Geometry check sheet. Reference: the model listing, model coordinates, mm. A direction names the side the tool comes from. Give positions to 0.01 mm unless a question says otherwise; leave off trailing zeros. Write each loop counter-clockwise with the first axis right and the second up, starting at its lowest first coordinate (ties: lowest second). Pieces come first, ordered by that corner, then holes. Notation, with made-up numbers: (-2.5, 9) -> (16.5, 9) arc R26 cw to (16.5, 47) -> close; hole circle Ø8 at (5.25, 16.5). An arc over 180 degrees is marked (long way). One line per item, written item: value.
from build123d import *

# Parameters (mm, degrees)
F0_W         = 88.9
F0_H         = 88.9
F0_W_2       = 57.15
F0_H_2       = 57.15
F1_DEPTH     = 177.8
F2_DEPTH     = 15.875
F3_R         = 3.429
F4_T1_DEPTH  = 57.15
F4_T3_DEPTH  = 57.15
F4_T9_DEPTH  = 97.975467434
F4_T13_DEPTH = 97.975467434
F4_T20_DEPTH = 97.975467434
F4_T24_DEPTH = 97.975467434
F4_T31_DEPTH = 97.975467434
F4_T35_DEPTH = 97.975467434
F4_T42_DEPTH = 97.975467434
F4_T46_DEPTH = 97.975467434


# Not quite as in the source:
# - a fillet or chamfer that OpenCascade refuses, or shapes differently, is made with other operations: its cross-section is extruded or revolved along the edge and cut away or added


with BuildPart() as f1:
    # F0 (on Front) → F1 (new body)
    with BuildSketch(Plane.XZ):
        Rectangle(F0_W, F0_H)
        Rectangle(F0_W_2, F0_H_2, mode=Mode.SUBTRACT)
    extrude(amount=-F1_DEPTH)

    # F0 (on Front) → F2 (join)
    with BuildSketch(Plane.XZ):
        Rectangle(F0_W, F0_H)
        Rectangle(F0_W_2, F0_H_2, mode=Mode.SUBTRACT)
        Rectangle(F0_W_2, F0_H_2)
    extrude(amount=-F2_DEPTH)

    # F3
    f3_edges = [f1.edges().sort_by_distance(p)[0] for p in [
        (44.45, 88.9, 44.45),
        (0, 0, 44.45),
        (44.45, 0, 0),
        (0, 0, -44.45),
        (44.45, 88.9, -44.45),
        (-44.45, 0, 0),
        (-44.45, 88.9, -44.45),
        (0, 177.8, 44.45),
        (-44.45, 88.9, 44.45),
        (-44.45, 177.8, 0),
        (0, 177.8, -44.45),
        (44.45, 177.8, 0),
    ]]
    fillet(f3_edges, radius=F3_R)

    # F4: chamfer of 15.875 on 4 edges, made by hand

    # F4_s2 → F4_t1 (cut)
    with BuildSketch(Plane.XY.offset(-28.575)):
        with BuildLine():
            Line((-44.8990128061, 178.2490128061), (-28.1259871939, 161.4759871939))
            Line((-28.1259871939, 161.4759871939), (-27.8084871939, 161.4759871939))
            ThreePointArc((-27.8084871939, 161.4759871939), (-28.2575, 169.637993597), (-28.2575, 177.8))
            Line((-28.2575, 177.8), (-28.575, 178.1175))
            ThreePointArc((-28.575, 178.1175), (-36.737006403, 178.1175), (-44.8990128061, 178.5665128061))
            Line((-44.8990128061, 178.5665128061), (-44.8990128061, 178.2490128061))
        make_face()
        with BuildLine():
            Line((44.8990128061, 178.2490128061), (28.1259871939, 161.4759871939))
            Line((28.1259871939, 161.4759871939), (27.8084871939, 161.4759871939))
            ThreePointArc((27.8084871939, 161.4759871939), (28.2575, 169.637993597), (28.2575, 177.8))
            Line((28.2575, 177.8), (28.575, 178.1175))
            ThreePointArc((28.575, 178.1175), (36.737006403, 178.1175), (44.8990128061, 178.5665128061))
            Line((44.8990128061, 178.5665128061), (44.8990128061, 178.2490128061))
        make_face()
    extrude(amount=F4_T1_DEPTH, mode=Mode.SUBTRACT)

    # F4_s4 → F4_t3 (cut)
    with BuildSketch(Plane.YZ.offset(-28.575)):
        with BuildLine():
            Line((178.2490128061, -44.8990128061), (161.4759871939, -28.1259871939))
            Line((161.4759871939, -28.1259871939), (161.4759871939, -27.8084871939))
            ThreePointArc((161.4759871939, -27.8084871939), (169.637993597, -28.2575), (177.8, -28.2575))
            Line((177.8, -28.2575), (178.1175, -28.575))
            ThreePointArc((178.1175, -28.575), (178.1175, -36.737006403), (178.5665128061, -44.8990128061))
            Line((178.5665128061, -44.8990128061), (178.2490128061, -44.8990128061))
        make_face()
        with BuildLine():
            Line((178.2490128061, 44.8990128061), (161.4759871939, 28.1259871939))
            Line((161.4759871939, 28.1259871939), (161.4759871939, 27.8084871939))
            ThreePointArc((161.4759871939, 27.8084871939), (169.637993597, 28.2575), (177.8, 28.2575))
            Line((177.8, 28.2575), (178.1175, 28.575))
            ThreePointArc((178.1175, 28.575), (178.1175, 36.737006403), (178.5665128061, 44.8990128061))
            Line((178.5665128061, 44.8990128061), (178.2490128061, 44.8990128061))
        make_face()
    extrude(amount=F4_T3_DEPTH, mode=Mode.SUBTRACT)


with BuildPart() as f4_tool7:
    # F4_s8 → F4_t9 (new body)
    with BuildSketch(Plane.XY.offset(-69.400467434)):
        with BuildLine():
            Line((-44.8990128061, 178.2490128061), (-28.1259871939, 161.4759871939))
            Line((-28.1259871939, 161.4759871939), (-27.8084871939, 161.4759871939))
            ThreePointArc((-27.8084871939, 161.4759871939), (-28.2575, 169.637993597), (-28.2575, 177.8))
            Line((-28.2575, 177.8), (-28.575, 178.1175))
            ThreePointArc((-28.575, 178.1175), (-36.737006403, 178.1175), (-44.8990128061, 178.5665128061))
            Line((-44.8990128061, 178.5665128061), (-44.8990128061, 178.2490128061))
        make_face()
    extrude(amount=F4_T9_DEPTH)

    split(bisect_by=Plane.XY.offset(-28.575), keep=Keep.BOTTOM)


with BuildPart() as f4_tool11:
    # F4_s12 → F4_t13 (new body)
    with BuildSketch(Plane.YZ.offset(28.575)):
        with BuildLine():
            Line((178.2490128061, -44.8990128061), (161.4759871939, -28.1259871939))
            Line((161.4759871939, -28.1259871939), (161.4759871939, -27.8084871939))
            ThreePointArc((161.4759871939, -27.8084871939), (169.637993597, -28.2575), (177.8, -28.2575))
            Line((177.8, -28.2575), (178.1175, -28.575))
            ThreePointArc((178.1175, -28.575), (178.1175, -36.737006403), (178.5665128061, -44.8990128061))
            Line((178.5665128061, -44.8990128061), (178.2490128061, -44.8990128061))
        make_face()
    extrude(amount=-F4_T13_DEPTH)

    split(bisect_by=Plane.YZ.offset(-28.575), keep=Keep.BOTTOM)


with BuildPart() as f4_tool7_1:
    add(f4_tool7.part)

    # F4_t15: intersect F4_tool11
    add(f4_tool11.part, mode=Mode.INTERSECT)


with BuildPart() as f1_1:
    add(f1.part)

    # F4_t5: cut F4_tool7
    add(f4_tool7_1.part, mode=Mode.SUBTRACT)


with BuildPart() as f4_tool18:
    # F4_s19 → F4_t20 (new body)
    with BuildSketch(Plane.XY.offset(-28.575)):
        with BuildLine():
            Line((-44.8990128061, 178.2490128061), (-28.1259871939, 161.4759871939))
            Line((-28.1259871939, 161.4759871939), (-27.8084871939, 161.4759871939))
            ThreePointArc((-27.8084871939, 161.4759871939), (-28.2575, 169.637993597), (-28.2575, 177.8))
            Line((-28.2575, 177.8), (-28.575, 178.1175))
            ThreePointArc((-28.575, 178.1175), (-36.737006403, 178.1175), (-44.8990128061, 178.5665128061))
            Line((-44.8990128061, 178.5665128061), (-44.8990128061, 178.2490128061))
        make_face()
    extrude(amount=F4_T20_DEPTH)

    split(bisect_by=Plane.XY.offset(28.575), keep=Keep.TOP)


with BuildPart() as f4_tool22:
    # F4_s23 → F4_t24 (new body)
    with BuildSketch(Plane.YZ.offset(-69.400467434)):
        with BuildLine():
            Line((178.2490128061, 44.8990128061), (161.4759871939, 28.1259871939))
            Line((161.4759871939, 28.1259871939), (161.4759871939, 27.8084871939))
            ThreePointArc((161.4759871939, 27.8084871939), (169.637993597, 28.2575), (177.8, 28.2575))
            Line((177.8, 28.2575), (178.1175, 28.575))
            ThreePointArc((178.1175, 28.575), (178.1175, 36.737006403), (178.5665128061, 44.8990128061))
            Line((178.5665128061, 44.8990128061), (178.2490128061, 44.8990128061))
        make_face()
    extrude(amount=F4_T24_DEPTH)

    split(bisect_by=Plane.YZ.offset(-28.575), keep=Keep.BOTTOM)


with BuildPart() as f4_tool18_1:
    add(f4_tool18.part)

    # F4_t26: intersect F4_tool22
    add(f4_tool22.part, mode=Mode.INTERSECT)


with BuildPart() as f1_2:
    add(f1_1.part)

    # F4_t16: cut F4_tool18
    add(f4_tool18_1.part, mode=Mode.SUBTRACT)


with BuildPart() as f4_tool29:
    # F4_s30 → F4_t31 (new body)
    with BuildSketch(Plane.XY.offset(28.575)):
        with BuildLine():
            Line((44.8990128061, 178.2490128061), (28.1259871939, 161.4759871939))
            Line((28.1259871939, 161.4759871939), (27.8084871939, 161.4759871939))
            ThreePointArc((27.8084871939, 161.4759871939), (28.2575, 169.637993597), (28.2575, 177.8))
            Line((28.2575, 177.8), (28.575, 178.1175))
            ThreePointArc((28.575, 178.1175), (36.737006403, 178.1175), (44.8990128061, 178.5665128061))
            Line((44.8990128061, 178.5665128061), (44.8990128061, 178.2490128061))
        make_face()
    extrude(amount=-F4_T31_DEPTH)

    split(bisect_by=Plane.XY.offset(-28.575), keep=Keep.BOTTOM)


with BuildPart() as f4_tool33:
    # F4_s34 → F4_t35 (new body)
    with BuildSketch(Plane.YZ.offset(69.400467434)):
        with BuildLine():
            Line((178.2490128061, -44.8990128061), (161.4759871939, -28.1259871939))
            Line((161.4759871939, -28.1259871939), (161.4759871939, -27.8084871939))
            ThreePointArc((161.4759871939, -27.8084871939), (169.637993597, -28.2575), (177.8, -28.2575))
            Line((177.8, -28.2575), (178.1175, -28.575))
            ThreePointArc((178.1175, -28.575), (178.1175, -36.737006403), (178.5665128061, -44.8990128061))
            Line((178.5665128061, -44.8990128061), (178.2490128061, -44.8990128061))
        make_face()
    extrude(amount=-F4_T35_DEPTH)

    split(bisect_by=Plane.YZ.offset(28.575), keep=Keep.TOP)


with BuildPart() as f4_tool29_1:
    add(f4_tool29.part)

    # F4_t37: intersect F4_tool33
    add(f4_tool33.part, mode=Mode.INTERSECT)


with BuildPart() as f1_3:
    add(f1_2.part)

    # F4_t27: cut F4_tool29
    add(f4_tool29_1.part, mode=Mode.SUBTRACT)


with BuildPart() as f4_tool40:
    # F4_s41 → F4_t42 (new body)
    with BuildSketch(Plane.YZ.offset(-28.575)):
        with BuildLine():
            Line((178.2490128061, 44.8990128061), (161.4759871939, 28.1259871939))
            Line((161.4759871939, 28.1259871939), (161.4759871939, 27.8084871939))
            ThreePointArc((161.4759871939, 27.8084871939), (169.637993597, 28.2575), (177.8, 28.2575))
            Line((177.8, 28.2575), (178.1175, 28.575))
            ThreePointArc((178.1175, 28.575), (178.1175, 36.737006403), (178.5665128061, 44.8990128061))
            Line((178.5665128061, 44.8990128061), (178.2490128061, 44.8990128061))
        make_face()
    extrude(amount=F4_T42_DEPTH)

    split(bisect_by=Plane.YZ.offset(28.575), keep=Keep.TOP)


with BuildPart() as f4_tool44:
    # F4_s45 → F4_t46 (new body)
    with BuildSketch(Plane.XY.offset(69.400467434)):
        with BuildLine():
            Line((44.8990128061, 178.2490128061), (28.1259871939, 161.4759871939))
            Line((28.1259871939, 161.4759871939), (27.8084871939, 161.4759871939))
            ThreePointArc((27.8084871939, 161.4759871939), (28.2575, 169.637993597), (28.2575, 177.8))
            Line((28.2575, 177.8), (28.575, 178.1175))
            ThreePointArc((28.575, 178.1175), (36.737006403, 178.1175), (44.8990128061, 178.5665128061))
            Line((44.8990128061, 178.5665128061), (44.8990128061, 178.2490128061))
        make_face()
    extrude(amount=-F4_T46_DEPTH)

    split(bisect_by=Plane.XY.offset(28.575), keep=Keep.TOP)


with BuildPart() as f4_tool40_1:
    add(f4_tool40.part)

    # F4_t48: intersect F4_tool44
    add(f4_tool44.part, mode=Mode.INTERSECT)


with BuildPart() as f1_4:
    add(f1_3.part)

    # F4_t38: cut F4_tool40
    add(f4_tool40_1.part, mode=Mode.SUBTRACT)


solid = f1_4.part
1) Mould release check, pull along X, two halves, no side actions. Record for faces 3 (the flat face through (-0.6, 169.46, 36.11)), 4 (the cylindrical face through (43.47, 1.03, 0.57)), 5 (the cylindrical face through (-43.47, 90.1, 43.42)), 6 (the flat face through (0.6, 169.46, -36.11)): released by +X, released by -X, zero draft, split by the parting line, or undercut.
Verdict:
face 3: undercut
face 4: released by +X
face 5: released by -X
face 6: undercut
2) Scan lines: probe 1 along Z at (x, y) = (18, 19.5) (3 decimals); probe 2 along X at (y, z) = (73.5, 41.5). Record each from-to range of solid material in increasing order.
Verdict:
probe 1: -44.45 to -28.575, 28.575 to 44.45
probe 2: -44.42 to 44.42
3) Sectioned sample at A-A on y = 129.5. Record the cut outline in (x, z) (3 decimals).
Verdict:
outline: (-44.45, -41.021) arc R3.429 ccw to (-41.021, -44.45) -> (41.021, -44.45) arc R3.429 ccw to (44.45, -41.021) -> (44.45, 41.021) arc R3.429 ccw to (41.021, 44.45) -> (-41.021, 44.45) arc R3.429 ccw to (-44.45, 41.021) -> close; hole (-28.575, -28.575) -> (28.575, -28.575) -> (28.575, 28.575) -> (-28.575, 28.575) -> close
4) Sectioned sample at C-C on x = 31.5. Record the cut outline in (y, z), plus the area to 3 significant figures.
Verdict:
outline: (0, -41.02) arc R3.43 ccw to (3.43, -44.45) -> (174.37, -44.45) arc R3.43 ccw to (176.8, -43.45) -> (164.85, -31.5) -> (164.85, 31.5) -> (176.8, 43.45) arc R3.43 ccw to (174.37, 44.45) -> (3.43, 44.45) arc R3.43 ccw to (0, 41.02) -> close
area: 14,800 mm^2
5) Sectioned sample at D-D on z = -23.5. Record the cut outline in (x, y) (3 decimals).
Verdict:
outline: (-44.45, 3.429) arc R3.429 ccw to (-41.021, 0) -> (41.021, 0) arc R3.429 ccw to (44.45, 3.429) -> (44.45, 174.371) arc R3.429 ccw to (43.446, 176.796) -> (28.575, 161.925) -> (28.575, 15.875) -> (-28.575, 15.875) -> (-28.575, 161.925) -> (-43.446, 176.796) arc R3.429 ccw to (-44.45, 174.371) -> close
6) Depth check by flat-ended pin: pin 1 Ø8 at (x, z) = (11, 32) entering from +Y. Enter the tip coordinate at first touch or a pass-through.
Verdict:
pin 1: y = 169.35
7) Sectioned sample at B-B on z = 34. Record the cut outline in (x, y), plus the area to 3 significant figures.
Verdict:
outline: (-44.45, 3.43) arc R3.43 ccw to (-41.02, 0) -> (41.02, 0) arc R3.43 ccw to (44.45, 3.43) -> (44.45, 174.37) arc R3.43 ccw to (43.45, 176.8) -> (34, 167.35) -> (-34, 167.35) -> (-43.45, 176.8) arc R3.43 ccw to (-44.45, 174.37) -> close
area: 15,000 mm^2
8) Tool access check on faces 1 (the flat face through (-28.575, 88, 0)), 2 (the cylindrical face through (0.57, 1.03, -43.47)). Record the directions out of +Z, -Z, +X, -X, +Y, -Y that give a thin tool (end or side, any length) a straight path to the whole face; none if there is none.
Verdict:
face 1: +Y
face 2: -Z, +X, -X, -Y
